```python
from build123d import *

# Parameters (mm, degrees)
SKETCH1_R           = 50
EXTRUDE1_DEPTH      = 38
EXTRUDE2_DEPTH      = 4
EXTRUDE2_DEPTH_BACK = 42
SKETCH2_R           = 12
SKETCH3_R           = 5
EXTRUDE3_DEPTH      = 77
SKETCH4_R           = 37
SKETCH4_R_2         = 12
EXTRUDE4_DEPTH      = 10
EXTRUDE6_START      = -10
SKETCH5_R           = 37
SKETCH5_R_2         = 12
EXTRUDE6_DEPTH      = 10
FILLET1_R           = 4
SKETCH6_R           = 1
EXTRUDE7_DEPTH      = 12


with BuildPart() as part:
    # Sketch1 → Extrude1 (new body)
    with BuildSketch(Plane(origin=(0, 0, 0), x_dir=(1, 0, 0), z_dir=(0, 1, 0))):
        with Locations(Location((0, 0, 0), (0, 0, 270))):
            Circle(SKETCH1_R)
    extrude(amount=EXTRUDE1_DEPTH)

    # Sketch2 → Extrude2 (add, two sides: drawn at the far end of the back side and taken through both)
    with BuildSketch(Plane.XZ.offset(-EXTRUDE2_DEPTH_BACK)):
        with Locations(Location((0, 0, 0), (0, 0, 270))):
            Circle(SKETCH2_R)
    extrude(amount=EXTRUDE2_DEPTH + EXTRUDE2_DEPTH_BACK)

    # Sketch3 → Extrude3 (cut)
    with BuildSketch(Plane.XZ.offset(4)):
        with Locations(Location((0, 0, 0), (0, 0, 270))):
            Circle(SKETCH3_R)
    extrude(amount=-EXTRUDE3_DEPTH, mode=Mode.SUBTRACT)

    # Sketch4 → Extrude4 (cut)
    with BuildSketch(Plane.XZ):
        with Locations(Location((0, 0, 0), (0, 0, 270))):
            Circle(SKETCH4_R)
        with Locations(Location((0, 0, 0), (0, 0, 270))):
            Circle(SKETCH4_R_2, mode=Mode.SUBTRACT)
    extrude(amount=-EXTRUDE4_DEPTH, mode=Mode.SUBTRACT)

    # Sketch5 → Extrude6 (cut)
    with BuildSketch(Plane(origin=(0, 38, 0), x_dir=(1, 0, 0), z_dir=(0, 1, 0)).offset(EXTRUDE6_START)):
        with Locations(Location((0, 0, 0), (0, 0, 90))):
            Circle(SKETCH5_R)
        with Locations(Location((0, 0, 0), (0, 0, 90))):
            Circle(SKETCH5_R_2, mode=Mode.SUBTRACT)
    extrude(amount=EXTRUDE6_DEPTH, mode=Mode.SUBTRACT)

    # Fillet1
    fillet1_edges = [part.edges().sort_by_distance(p)[0] for p in [
        (0, 0, -50),
        (0, 38, -50),
    ]]
    fillet(fillet1_edges, radius=FILLET1_R)

    # Sketch6 → Extrude7 (cut)
    with BuildSketch(Plane.XY):
        with Locations(Location((0, 36, 0), (0, 0, 90))):
            Circle(SKETCH6_R)
    extrude(amount=-EXTRUDE7_DEPTH, mode=Mode.SUBTRACT)


solid = part.part
```
Source: CAD feature listing. Evaluate the final solid. Frame: model axes, mm. A direction names the side the tool comes from. Round coordinates to 2 decimals unless told otherwise and drop trailing zeros. Order: outer loops, then holes, each group sorted by start corner. A loop starts at its lowest first (then second) coordinate and runs counter-clockwise, first axis right, second up. Notation, with made-up numbers: (10.25, 37) -> (22.25, 37) arc R13 ccw to (22.25, 58) -> close; hole circle Ø8 at (5, -17.5). An arc over 180 degrees is marked (long way). One line per item, written item: value. Start each with the question number.
Q1. Access query for faces 1 (the cylindrical face through (-4.88, 18.68, 1.08)), 2 (the cylindrical face through (3.604, 35.098, -11.446)), 3 (the cylindrical face through (-14.17, 4.93, -34.18)). Directions: +Z, -Z, +X, -X, +Y, -Y. A direction counts if a zero-diameter tool reaches every point of the face in a straight line with its end or side. Return the directions, or none.
Q2. Pin query (flat end, axial travel): pin 1 (10 mm diameter, centred on x = -11, y = 11.5, fed in from +Z); pin 2 (1.5 mm diameter, centred on y = 29.5, z = -4, fed in from -X); pin 3 (5 mm diameter, centred on x = 2.5, z = -19, fed in from +Y); pin 4 (9 mm diameter, centred on x = 0, z = 0, fed in from -Y). Return the tip coordinate at first contact, or that it passes through.
Q3. Draft query along X for faces 4 (the cylindrical face through (14.17, 32.93, -34.18)), 5 (the cylindrical face through (15.02, 18.79, 47.69)), 6 (the flat face through (21, 0, -31)). Return one class per face: pulls with the +X half, pulls with the -X half, needs draft (parallel to the pull), parting line crosses it, or undercut.
Q4. Section query B-B (y = 31.5). Return the cut outline in (x, z).
Q5. Section query A-A (z = 0). Return the cut outline in (x, y), plus the area to 3 significant figures.
Q6. Material intervals for probe 1 along X at (y, z) = (8.25, 0); probe 2 along X at (y, z) = (21.5, 0); probe 3 along X at (y, z) = (36, -6.5), sorted ascending.
Q7. Section query C-C (y = 14.5). Return the cut outline in (x, z).
Findings below:
1. face 1: +Y, -Y
1. face 2: +Y
1. face 3: -Y
2. pin 1: z = 49.64
2. pin 2: x = -49.89
2. pin 3: y = 28
2. pin 4: through
3. face 4: undercut
3. face 5: parting line crosses it
3. face 6: needs draft
4. outline: circle Ø100 at (0, 0); circle Ø24 at (0, 0); hole circle Ø74 at (0, 0); hole circle Ø10 at (0, 0)
5. outline: (-50, 4) arc R4 ccw to (-46, 0) -> (-37, 0) -> (-37, 10) -> (-12, 10) -> (-12, -4) -> (-5, -4) -> (-5, 42) -> (-12, 42) -> (-12, 28) -> (-37, 28) -> (-37, 38) -> (-46, 38) arc R4 ccw to (-50, 34) -> close; (5, -4) -> (12, -4) -> (12, 10) -> (37, 10) -> (37, 0) -> (46, 0) arc R4 ccw to (50, 4) -> (50, 34) arc R4 ccw to (46, 38) -> (37, 38) -> (37, 28) -> (12, 28) -> (12, 42) -> (5, 42) -> close
5. area: 2,520 mm²
6. probe 1: -50 to -37, -12 to -5, 5 to 12, 37 to 50
6. probe 2: -50 to -5, 5 to 50
6. probe 3: -49.04 to -36.42, -10.09 to -1, 1 to 10.09, 36.42 to 49.04
7. outline: circle Ø100 at (0, 0); hole circle Ø10 at (0, 0)
